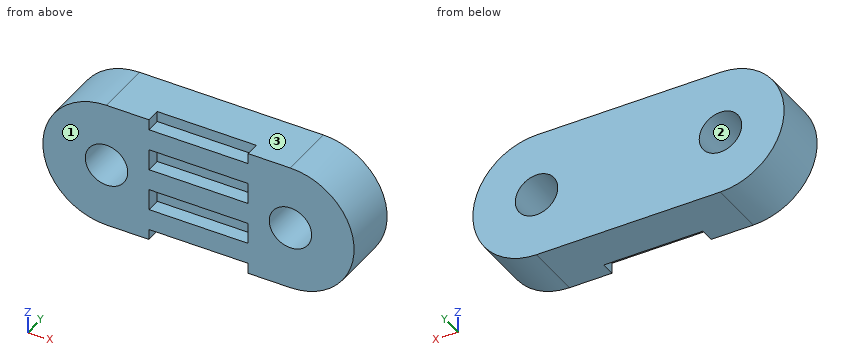
```python
from build123d import *

# Parameters (mm, degrees)
SKETCH1_R      = 1.5
EXTRUDE1_DEPTH = 4
SKETCH2_W      = 7
SKETCH2_H      = 0.75
SKETCH2_H_2    = 1.5
EXTRUDE4_DEPTH = 1


with BuildPart() as part:
    # Sketch1 → Extrude1 (new body)
    with BuildSketch(Plane(origin=(0, 0, 0), x_dir=(1, 0, 0), z_dir=(0, 1, 0))):
        with BuildLine():
            Line((-6.5, 4.5), (6.5, 4.5))
            ThreePointArc((6.5, 4.5), (11, 0), (6.5, -4.5))
            Line((6.5, -4.5), (-6.5, -4.5))
            ThreePointArc((-6.5, -4.5), (-11, 0), (-6.5, 4.5))
        make_face()
        with Locations((6.5, 0)):
            Circle(SKETCH1_R, mode=Mode.SUBTRACT)
        with Locations((-6.5, 0)):
            Circle(SKETCH1_R, mode=Mode.SUBTRACT)
    extrude(amount=EXTRUDE1_DEPTH)

    # Sketch2 → Extrude4 (cut)
    with BuildSketch(Plane.XZ):
        with Locations((0, -4.125)):
            Rectangle(SKETCH2_W, SKETCH2_H)
        with Locations((0, -1.5)):
            Rectangle(SKETCH2_W, SKETCH2_H_2)
        with Locations((0, 1.5)):
            Rectangle(SKETCH2_W, SKETCH2_H_2)
        with Locations((0, 4.125)):
            Rectangle(SKETCH2_W, SKETCH2_H)
    extrude(amount=-EXTRUDE4_DEPTH, mode=Mode.SUBTRACT)


solid = part.part
```
Work out the finished part from the listing and answer in its coordinate system (mm). Face numbers are marked on the shaded views. Coordinates: 2 decimals unless noted, no trailing zeros. Loops run counter-clockwise (first coordinate to the right, second up) from the corner with the lowest first, then second, coordinate; pieces in that order, holes last.
1) Flat-ended cylindrical pins translate along their axes: pin 1 (0.5 mm diameter, centred on y = 0.5, z = 1.5, fed in from -X); pin 2 (1.8 mm diameter, centred on x = -6.5, z = 0, fed in from -Y); pin 3 (0.8 mm diameter, centred on x = 1, y = 0.5, fed in from +Z); pin 4 (2 mm diameter, centred on x = 8, y = 2.5, fed in from +Z). Find the tip coordinate at first contact, or state that the pin passes through.
Results:
pin 1: stops at x = -10.82
pin 2: passes through
pin 3: stops at z = 3.75
pin 4: stops at z = 4.47
2) Section D-D (z = -4) is taken. Give the vertices of the cut face in (x, y).
Results:
outline: (-8.56, 0) - (-3.5, 0) - (-3.5, 1) - (3.5, 1) - (3.5, 0) - (8.56, 0) - (8.56, 4) - (-8.56, 4) - close
3) Section A-A (z = 0) is taken. Give the vertices of the cut face in (x, y), plus the area to 3 significant figures.
Results:
outline: (-11, 0) - (-8, 0) - (-8, 4) - (-11, 4) - close; (-5, 0) - (5, 0) - (5, 4) - (-5, 4) - close; (8, 0) - (11, 0) - (11, 4) - (8, 4) - close
area: 64.0 mm2
4) For a pull along Z with two mould halves and no side action, classify the marked faces 1, 2 and 3 as +Z half, -Z half, draft (parallel to the pull), parting line (faces both ways), or undercut.
Results:
face 1: draft
face 2: undercut
face 3: +Z half
5) Section C-C (x = -1.5) is taken. Give the vertices of the cut face in (y, z).
Results:
outline: (0, -3.75) - (1, -3.75) - (1, -4.5) - (4, -4.5) - (4, 4.5) - (1, 4.5) - (1, 3.75) - (0, 3.75) - (0, 2.25) - (1, 2.25) - (1, 0.75) - (0, 0.75) - (0, -0.75) - (1, -0.75) - (1, -2.25) - (0, -2.25) - close
6) Section B-B (y = 3.65) is taken. Give the vertices of the cut face in (x, z).
Results:
outline: (-6.5, -4.5) - (6.5, -4.5) arc R4.5 ccw to (6.5, 4.5) - (-6.5, 4.5) arc R4.5 ccw to start; hole circle Ø3 at (-6.5, 0); hole circle Ø3 at (6.5, 0)
7) Consider probe 1 along Z at (x, y) = (1.5, 0.6); probe 2 along X at (y, z) = (1.75, 0); probe 3 along Z at (x, y) = (-6.5, 0.95). Determine where each line is inside the solid, lowest interval first.
Results:
probe 1: z = -3.75 to -2.25, -0.75 to 0.75, 2.25 to 3.75
probe 2: x = -11 to -8, -5 to 5, 8 to 11
probe 3: z = -4.5 to -1.5, 1.5 to 4.5
